```python
from build123d import *

# Parameters (mm, degrees)
SIDE_BOSS_EXTRUDE1_DEPTH                 = 4
SIDE_BOSS_EXTRUDE1_DEPTH_BACK            = 4
SKETCH3_W                                = 50
SKETCH3_H                                = 8
SOCKET_TOP_AND_BOTTOM_CUT_EXTRUDE1_DEPTH = 8
SKETCH4_R                                = 1.5
MOUNTING_HOLES_TOP_CUT_EXTRUDE2_DEPTH    = 10
MOUNTING_START                           = -10
SKETCH5_R                                = 1.5
MOUNTING_HOLES_BOTTOM_CUT_EXTRUDE3_DEPTH = 10


with BuildPart() as part:
    # Sketch2 → Side Boss-Extrude1 (new, two sides: drawn at the far end of the back side and taken through both)
    with BuildSketch(Plane.XY.offset(-SIDE_BOSS_EXTRUDE1_DEPTH_BACK)):
        Polygon((-86.592068141, 50), (86.592068141, 50), (91.670882932, 0), (-91.670882932, 0), align=None)
    extrude(amount=SIDE_BOSS_EXTRUDE1_DEPTH + SIDE_BOSS_EXTRUDE1_DEPTH_BACK)

    # Sketch3 → Socket Top And Bottom Cut-Extrude1 (cut)
    with BuildSketch(Plane.XY.offset(4)):
        with Locations((0, 4)):
            Rectangle(SKETCH3_W, SKETCH3_H)
        Polygon((25, 42), (0, 42), (-25, 42), (-25, 50), (25, 50), align=None)
    extrude(amount=-SOCKET_TOP_AND_BOTTOM_CUT_EXTRUDE1_DEPTH, mode=Mode.SUBTRACT)

    # Sketch4 → Mounting Holes Top Cut-Extrude2 (cut)
    with BuildSketch(Plane(origin=(0, 42, 0), x_dir=(1, 0, 0), z_dir=(0, 1, 0))):
        with Locations(Location((20, 0, 0), (0, 0, 180))):
            Circle(SKETCH4_R)
        with Locations(Location((-20, 0, 0), (0, 0, 180))):
            Circle(SKETCH4_R)
    extrude(amount=-MOUNTING_HOLES_TOP_CUT_EXTRUDE2_DEPTH, mode=Mode.SUBTRACT)

    # Sketch5 → Mounting Holes Bottom Cut-Extrude3 (cut)
    with BuildSketch(Plane.XZ.offset(-8).offset(MOUNTING_START)):
        with Locations(Location((20, 0, 0), (0, 0, 180))):
            Circle(SKETCH5_R)
        with Locations(Location((-20, 0, 0), (0, 0, 180))):
            Circle(SKETCH5_R)
    extrude(amount=MOUNTING_HOLES_BOTTOM_CUT_EXTRUDE3_DEPTH, mode=Mode.SUBTRACT)


solid = part.part
```
Read the model definition and answer for the solid it produces. Units are mm, in the model's axes. A direction names the side the tool comes from. Give positions to 0.01 mm unless a question says otherwise; leave off trailing zeros. Order: outer loops, then holes, each group sorted by start corner. A loop starts at its lowest first (then second) coordinate and runs counter-clockwise, first axis right, second up. Notation, with made-up numbers: (-24.75, 16.25) -> (15.25, 16.25) arc R20 ccw to (15.25, 36.25) -> close; hole circle Ø5 at (-33.5, 12). An arc over 180 degrees is marked (long way). One line per item, written item: value. Start each with the question number.
(1) The part is cut by section B-B (z = 0). Determine the outline of the cut face in (x, y), and give its area (3 significant figures).
(2) Straight lines are drawn through the part: L1, parallel to Z at x = 20, y = 15; L2, parallel to Y at x = -19.5, z = -2.5; L3, parallel to X at y = 41, z = -3.5. For each, find the intervals that lie inside material, in ascending order.
(3) The part is cut by section D-D (x = 1.5). Determine the outline of the cut face in (y, z), and give its area (3 significant figures).
(4) Flat-ended cylindrical pins translate along their axes: P1, Ø3.5, axis at x = -20.5, z = 0.5, coming from the -Y side; P2, Ø1.5, axis at x = 20.5, z = 0.5, coming from the +Y side; P3, Ø3.5, axis at x = -20, z = 0, coming from the +Y side. Find the tip coordinate at first contact, or state that the pin passes through.
(5) A tool of negligible diameter and unlimited length cuts with its end or side. For faces 1 (the flat face through (20, 18, 0)), 2 (the flat face through (25, 4, 0)), 3 (the cylindrical face through (21.5, 37.07, 0.07)), from which of +Z, -Z, +X, -X, +Y, -Y can it reach the whole face along a straight path? Write none if from no direction.
(6) For a pull along X with two mould halves and no side action, classify faces 4 (the flat face through (1, 25, -4)), 5 (the flat face through (-20, 32, 0)), 6 (the flat face through (89.1, 25.3, -0.1)) as released by +X, released by -X, zero draft, split by the parting line, or undercut.
(7) The part is cut by section C-C (y = 14). Determine the outline of the cut face in (x, z).
(8) The part is cut by section A-A (y = 45.5). Determine the outline of the cut face in (x, z).
Taken from the geometry:
1. outline: (-91.67, 0) -> (-25, 0) -> (-25, 8) -> (-21.5, 8) -> (-21.5, 18) -> (-18.5, 18) -> (-18.5, 8) -> (18.5, 8) -> (18.5, 18) -> (21.5, 18) -> (21.5, 8) -> (25, 8) -> (25, 0) -> (91.67, 0) -> (86.59, 50) -> (25, 50) -> (25, 42) -> (21.5, 42) -> (21.5, 32) -> (18.5, 32) -> (18.5, 42) -> (-18.5, 42) -> (-18.5, 32) -> (-21.5, 32) -> (-21.5, 42) -> (-25, 42) -> (-25, 50) -> (-86.59, 50) -> close
1. area: 7,990 mm^2
2. L1: -4 to -1.5, 1.5 to 4
2. L2: 8 to 42
2. L3: -87.51 to 87.51
3. outline: (8, -4) -> (42, -4) -> (42, 4) -> (8, 4) -> close
3. area: 272 mm^2
4. P1: y = 8
4. P2: y = 32
4. P3: y = 42
5. face 1: -Y
5. face 2: +Z, -Z, -Y
5. face 3: +Y
6. face 4: zero draft
6. face 5: undercut
6. face 6: released by +X
7. outline: (-90.25, -4) -> (90.25, -4) -> (90.25, 4) -> (-90.25, 4) -> close; hole circle Ø3 at (-20, 0); hole circle Ø3 at (20, 0)
8. outline: (-87.05, -4) -> (-25, -4) -> (-25, 4) -> (-87.05, 4) -> close; (25, -4) -> (87.05, -4) -> (87.05, 4) -> (25, 4) -> close
